Design review of the part built by this model. Coordinates are the model's own, in mm. A direction names the side the tool comes from. Coordinates: 2 decimals unless noted, no trailing zeros. Loops run counter-clockwise (first coordinate to the right, second up) from the corner with the lowest first, then second, coordinate; pieces in that order, holes last. Notation, with made-up numbers: (38.5, 24) - (56.5, 24) arc R34 ccw to (56.5, 57) - close; hole circle Ø7 at (66.25, 43). An arc over 180 degrees is marked (long way). Use one line per item in the form item = value. Start each with the question number.
(1) Add section A-A (x = 0). State the section outline as (y, z) points, plus the area to 3 significant figures.
(2) Add section D-D (x = -30). State the section outline as (y, z) points.
(3) Clearance check with flat-ended pins moving along their axes: pin 1 Ø1 at (x, y) = (2, -9) entering from +Z; pin 2 Ø10 at (x, y) = (14, -9.5) entering from +Z. State where each tip first meets the part, or that it passes through.
(4) Add section C-C (y = 16.5). State the section outline as (x, z) points, plus the area to 3 significant figures.
(5) The part is to be moulded in two halves that separate along X. For faces 1 (the face through (-37.685, 13, 0)), 2 (the face through (17.868, -0.356, 5.627)), 3 (the face through (-5.712, -12.522, -25.723)), 4 (the face through (37.685, 13, 0)), say which applies: pulls with the +X half, pulls with the -X half, needs draft (parallel to the pull), parting line crosses it, or undercut.
(6) For L1, parallel to X at y = 6.5, z = 0; L2, parallel to Z at x = 0, y = 1; L3, parallel to Z at x = 0, y = -8, list the stretches that pass through material, from the lowest coordinate up.
(7) Tool access review of faces 5 (the face through (-1, 13, -32.763)), 6 (the face through (-26, 0, 8)): name each direction out of +Z, -Z, +X, -X, +Y, -Y from which nothing blocks a thin tool from reaching the whole face with its end or side.
(8) Add section B-B (z = 0). State the section outline as (x, y) points.
```python
from build123d import *

# Parameters (mm, degrees)
F0_W     = 75.369708
F0_H     = 65.526642
F1_DEPTH = 25.4
F2_R     = 26.349112
F3_DEPTH = 25.4
F4_R     = 18.733501
F5_DEPTH = 25.401
F6_DEPTH = 25.401


with BuildPart() as f1:
    # F0 (on Front) → F1 (new body)
    with BuildSketch(Plane.XZ):
        Rectangle(F0_W, F0_H)
    extrude(amount=-F1_DEPTH)

    # F2 (on Front) → F3 (join)
    with BuildSketch(Plane.XZ):
        Circle(F2_R)
    extrude(amount=F3_DEPTH)

    # F4 (on Front) → F5 (cut, through all)
    with BuildSketch(Plane.XZ):
        Circle(F4_R)
    extrude(amount=F5_DEPTH, mode=Mode.SUBTRACT)

    # F4 (on Front) → F6 (cut, through all)
    with BuildSketch(Plane.XZ):
        Circle(F4_R)
    extrude(amount=-F6_DEPTH, mode=Mode.SUBTRACT)


solid = f1.part
```
Computed values:
q1.outline = (-25.4, -26.35) - (0, -26.35) - (0, -32.76) - (25.4, -32.76) - (25.4, -18.73) - (-25.4, -18.73) - close; (-25.4, 18.73) - (25.4, 18.73) - (25.4, 32.76) - (0, 32.76) - (0, 26.35) - (-25.4, 26.35) - close
q1.area = 1,100 mm^2
q2.outline = (0, -32.76) - (25.4, -32.76) - (25.4, 32.76) - (0, 32.76) - close
q3.pin_1 = 26.31
q3.pin_2 = 24.76
q4.outline = (-37.68, -32.76) - (37.68, -32.76) - (37.68, 32.76) - (-37.68, 32.76) - close; hole circle Ø37.47 at (0, 0)
q4.area = 3,840 mm^2
q5.face_1 = pulls with the -X half
q5.face_2 = undercut
q5.face_3 = parting line crosses it
q5.face_4 = pulls with the +X half
q6.L1 = -37.68 to -18.73, 18.73 to 37.68
q6.L2 = -32.76 to -18.73, 18.73 to 32.76
q6.L3 = -26.35 to -18.73, 18.73 to 26.35
q7.face_5 = -Z, +X, -X, +Y, -Y
q7.face_6 = -Y
q8.outline = (-37.68, 0) - (-26.35, 0) - (-26.35, -25.4) - (-18.73, -25.4) - (-18.73, 25.4) - (-37.68, 25.4) - close; (18.73, -25.4) - (26.35, -25.4) - (26.35, 0) - (37.68, 0) - (37.68, 25.4) - (18.73, 25.4) - close
